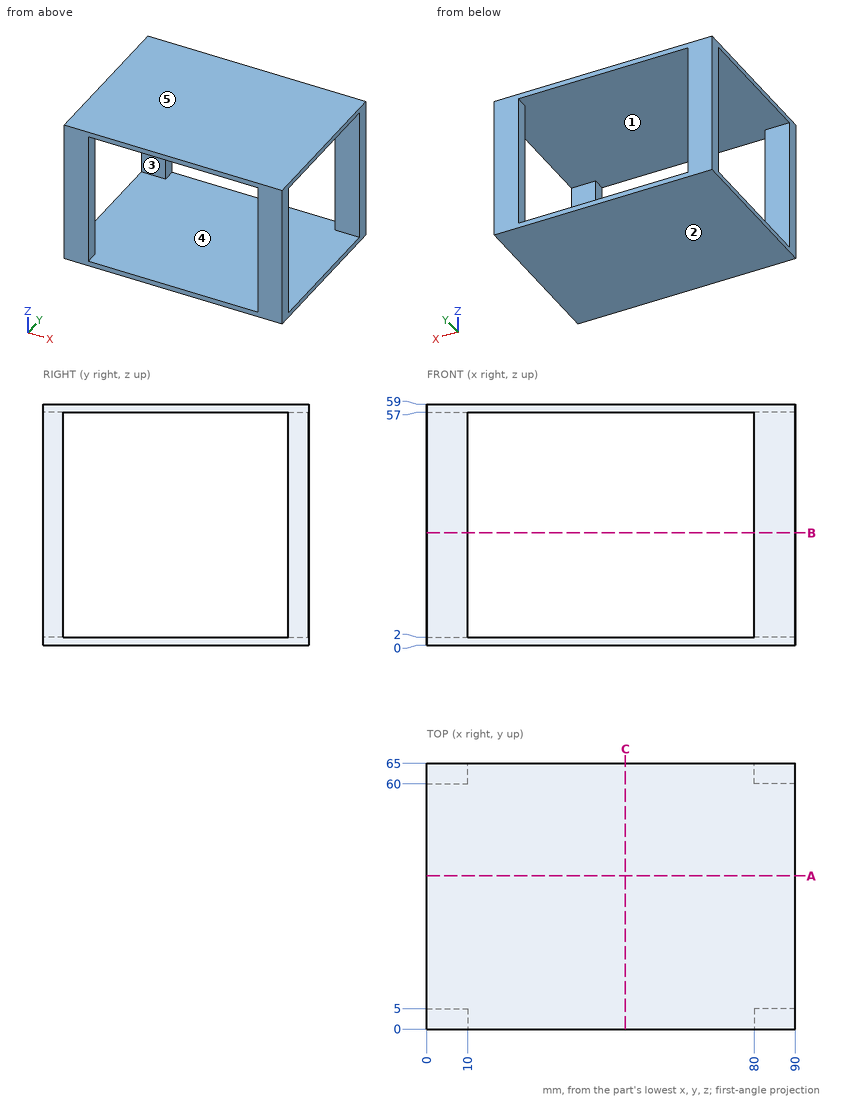
Drawing for the job (mm, zero at the part's lowest x, y, z). A direction names the side the tool comes from. Coordinates: 2 decimals unless noted, no trailing zeros. Order: outer loops, then holes, each group sorted by start corner. A loop starts at its lowest first (then second) coordinate and runs counter-clockwise, first axis right, second up. Notation, with made-up numbers: (-9.75, 66.25) - (14.25, 66.25) arc R26 cw to (14.25, 99.25) - close; hole circle Ø10 at (44.25, -34). An arc over 180 degrees is marked (long way). Use a Markdown table: item, result. Add a question column.
(1) Pull direction X, two halves, no side cores. Call the marked faces 1 and 2: +X half, -X half, draft (parallel to the pull), parting line (faces both ways), or undercut.
(2) Drill centre lines: line 1 along Z through (x, y) = (41.5, 60.5); line 2 along X through (y, z) = (61.5, 21). Where is each one in solid material? Low to high. Write a range as [from, to].
(3) Saw through at C-C (x = 48.5). Give the cut face in (y, z).
(4) Saw through at A-A (y = 37.5). Give the cut face in (x, z).
(5) Saw through at B-B (z = 27.5). Give the cut face in (x, y).
(6) Which spindle directions (+Z, -Z, +X, -X, +Y, -Y) get a long thin tool onto all of the face, cutting with end or side? Do the marked faces 3, 4 and 5. Say none if no direction does.
Solved:
| question | item | result |
|---|---|---|
| 1 | face 1 | undercut |
| 1 | face 2 | draft |
| 2 | line 1 | z = [0, 2], [57, 59] |
| 2 | line 2 | x = [0, 10], [80, 90] |
| 3 | outline | (0, 0) - (65, 0) - (65, 2) - (0, 2) - close; (0, 57) - (65, 57) - (65, 59) - (0, 59) - close |
| 4 | outline | (0, 0) - (90, 0) - (90, 2) - (0, 2) - close; (0, 57) - (90, 57) - (90, 59) - (0, 59) - close |
| 5 | outline | (0, 0) - (10, 0) - (10, 5) - (0, 5) - close; (0, 60) - (10, 60) - (10, 65) - (0, 65) - close; (80, 0) - (90, 0) - (90, 5) - (80, 5) - close; (80, 60) - (90, 60) - (90, 65) - (80, 65) - close |
| 6 | face 3 | +X, -X |
| 6 | face 4 | none |
| 6 | face 5 | +Z, +X, -X, +Y, -Y |
